The listing builds one solid part. Answer for the finished solid, in the listing's coordinates (mm). Face numbers are marked on the shaded views. A direction names the side the tool comes from. Round coordinates to 2 decimals unless told otherwise and drop trailing zeros. Loops run counter-clockwise (first coordinate to the right, second up) from the corner with the lowest first, then second, coordinate; pieces in that order, holes last. Notation, with made-up numbers: (66, 78) -> (76, 78) arc R20 ccw to (76, 108) -> close; hole circle Ø7 at (4, -2). An arc over 180 degrees is marked (long way). Write each question's results on one line, items separated by ' | '. Start each with the question number.
(1) The part is cut by section C-C (y = 2). Count the separate pieces of the cut face and the enclosed holes in it, plus the area to 3 significant figures.
(2) Flat-ended cylindrical pins translate along their axes: pin 1 (1.8 mm diameter, centred on x = 52.5, y = 2.5, fed in from -Z); pin 2 (4 mm diameter, centred on y = 10, z = 75, fed in from +X); pin 3 (6.5 mm diameter, centred on x = 52.5, y = 2, fed in from +Z). Find the tip coordinate at first contact, or state that the pin passes through.
(3) The part is cut by section B-B (z = 18.5). Determine the outline of the cut face in (x, y), plus the area to 3 significant figures.
(4) Straight lines are drawn through the part: probe 1 along Z at (x, y) = (-23.5, 1.25); probe 2 along X at (y, z) = (7.5, 64.5); probe 3 along Z at (x, y) = (53, 14.5). For each, find the intervals that lie inside material, in ascending order.
(5) Determine the mould class of the marked faces 1, 2, 3 and 4 for opening direction Z: released by +Z, released by -Z, zero draft, split by the parting line, or undercut.
(6) For the marked faces 5 and 6, determine the directions among +Z, -Z, +X, -X, +Y, -Y from which every point of the face is accessible in a straight line to the end or side of a thin tool.
(7) The part is cut by section A-A (x = 0). Determine the outline of the cut face in (y, z), plus the area to 3 significant figures.
```python
from build123d import *

# Parameters (mm, degrees)
BOSS_EXTRUDE1_DEPTH     = 16
SKETCH2_R               = 2.65
CUT_EXTRUDE1_DEPTH      = 20
CUT_EXTRUDE2_DEPTH      = 111.136478545
CUT_EXTRUDE2_DEPTH_BACK = 111.136478545
CUT_EXTRUDE3_DEPTH      = 111.136478545
CUT_EXTRUDE3_DEPTH_BACK = 111.136478545
SKETCH4_R               = 3.1
CUT_EXTRUDE4_DEPTH      = 111.136478545
CUT_EXTRUDE4_DEPTH_BACK = 6


with BuildPart() as part:
    # Sketch1 → Boss-Extrude1 (new body)
    with BuildSketch(Plane(origin=(0, 0, 0), x_dir=(1, 0, 0), z_dir=(0, 1, 0))):
        with BuildLine():
            Line((-44.75, 10.2375), (44.75, 10.2375))
            ThreePointArc((44.75, 10.2375), (57.301145366, 5.038645366), (62.5, -7.5125))
            Line((62.5, -7.5125), (62.5, -71.5125))
            ThreePointArc((62.5, -71.5125), (57.301145366, -84.063645366), (44.75, -89.2625))
            Line((44.75, -89.2625), (-44.75, -89.2625))
            ThreePointArc((-44.75, -89.2625), (-57.301145366, -84.063645366), (-62.5, -71.5125))
            Line((-62.5, -71.5125), (-62.5, -7.5125))
            ThreePointArc((-62.5, -7.5125), (-57.301145366, 5.038645366), (-44.75, 10.2375))
        make_face()
        with BuildLine():
            Line((-47.5, -7.5125), (-47.5, -71.5125))
            ThreePointArc((-47.5, -71.5125), (-46.694543648, -73.457043648), (-44.75, -74.2625))
            Line((-44.75, -74.2625), (44.75, -74.2625))
            ThreePointArc((44.75, -74.2625), (46.694543648, -73.457043648), (47.5, -71.5125))
            Line((47.5, -71.5125), (47.5, -7.5125))
            ThreePointArc((47.5, -7.5125), (46.694543648, -5.567956352), (44.75, -4.7625))
            Line((44.75, -4.7625), (-44.75, -4.7625))
            ThreePointArc((-44.75, -4.7625), (-46.694543648, -5.567956352), (-47.5, -7.5125))
        make_face(mode=Mode.SUBTRACT)
    extrude(amount=BOSS_EXTRUDE1_DEPTH)

    # Sketch2 → Cut-Extrude1 (cut)
    with BuildSketch(Plane.XY.offset(4.7625)):
        with Locations((0, 10.721875)):
            Circle(SKETCH2_R)
    extrude(amount=-CUT_EXTRUDE1_DEPTH, mode=Mode.SUBTRACT)

    # Sketch3 → Cut-Extrude2 (cut, two sides: drawn at the far end of the back side and taken through both)
    with BuildSketch(Plane(origin=(0, 0, 0), x_dir=(1, 0, 0), z_dir=(0, 1, 0)).offset(-CUT_EXTRUDE2_DEPTH_BACK)):
        with BuildLine():
            Line((-47.7, -7.5125), (-47.7, -71.5125))
            ThreePointArc((-47.7, -71.5125), (-46.835965004, -73.598465004), (-44.75, -74.4625))
            Line((-44.75, -74.4625), (44.75, -74.4625))
            ThreePointArc((44.75, -74.4625), (46.835965004, -73.598465004), (47.7, -71.5125))
            Line((47.7, -71.5125), (47.7, -7.5125))
            ThreePointArc((47.7, -7.5125), (46.835965004, -5.426534996), (44.75, -4.5625))
            Line((44.75, -4.5625), (-44.75, -4.5625))
            ThreePointArc((-44.75, -4.5625), (-46.835965004, -5.426534996), (-47.7, -7.5125))
        make_face()
        with BuildLine():
            Line((-44.75, -74.2625), (44.75, -74.2625))
            ThreePointArc((44.75, -74.2625), (46.694543648, -73.457043648), (47.5, -71.5125))
            Line((47.5, -71.5125), (47.5, -7.5125))
            ThreePointArc((47.5, -7.5125), (46.694543648, -5.567956352), (44.75, -4.7625))
            Line((44.75, -4.7625), (-44.75, -4.7625))
            ThreePointArc((-44.75, -4.7625), (-46.694543648, -5.567956352), (-47.5, -7.5125))
            Line((-47.5, -7.5125), (-47.5, -71.5125))
            ThreePointArc((-47.5, -71.5125), (-46.694543648, -73.457043648), (-44.75, -74.2625))
        make_face(mode=Mode.SUBTRACT)
    extrude(amount=CUT_EXTRUDE2_DEPTH + CUT_EXTRUDE2_DEPTH_BACK, mode=Mode.SUBTRACT)

    # Sketch4 → Cut-Extrude3 (cut, two sides: drawn at the far end of the back side and taken through both)
    with BuildSketch(Plane.XZ.offset(-CUT_EXTRUDE3_DEPTH_BACK)):
        with Locations(Location((-51.997844507, 78.760344507, 0), (0, 0, 270))):
            Circle(SKETCH4_R)
        with Locations(Location((51.997844507, 78.760344507, 0), (0, 0, 270))):
            Circle(SKETCH4_R)
        with Locations(Location((51.997844507, 0.264655493, 0), (0, 0, 270))):
            Circle(SKETCH4_R)
        with Locations(Location((-51.997844507, 0.264655493, 0), (0, 0, 270))):
            Circle(SKETCH4_R)
    extrude(amount=CUT_EXTRUDE3_DEPTH + CUT_EXTRUDE3_DEPTH_BACK, mode=Mode.SUBTRACT)

    # Sketch5 → Cut-Extrude4 (cut, two sides: drawn at the far end of the back side and taken through both)
    with BuildSketch(Plane.XZ.offset(-CUT_EXTRUDE4_DEPTH_BACK)):
        Polygon((-46.108871761, 78.760344507), (-49.053358134, 83.860344507), (-54.94233088, 83.860344507), (-57.886817253, 78.760344507), (-54.94233088, 73.660344507), (-49.053358134, 73.660344507), align=None)
        Polygon((57.886817253, 78.760344507), (54.94233088, 83.860344507), (49.053358134, 83.860344507), (46.108871761, 78.760344507), (49.053358134, 73.660344507), (54.94233088, 73.660344507), align=None)
        Polygon((57.886817253, 0.264655493), (54.94233088, 5.364655493), (49.053358134, 5.364655493), (46.108871761, 0.264655493), (49.053358134, -4.835344507), (54.94233088, -4.835344507), align=None)
        Polygon((-46.108871761, 0.264655493), (-49.053358134, 5.364655493), (-54.94233088, 5.364655493), (-57.886817253, 0.264655493), (-54.94233088, -4.835344507), (-49.053358134, -4.835344507), align=None)
    extrude(amount=CUT_EXTRUDE4_DEPTH + CUT_EXTRUDE4_DEPTH_BACK, mode=Mode.SUBTRACT)


solid = part.part
```
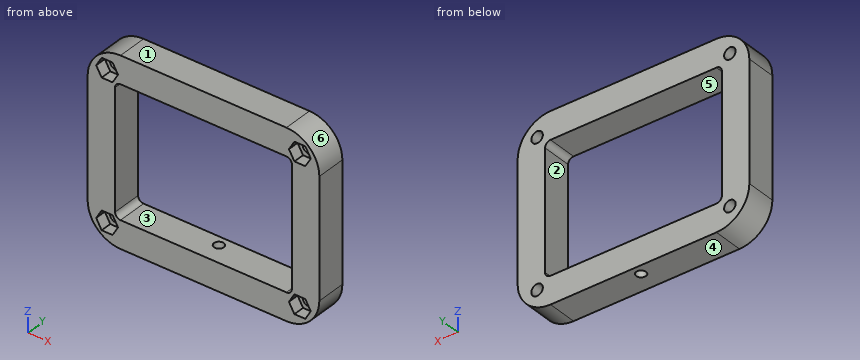
Checked values:
1) separate pieces: 1 | enclosed holes: 5 | area: 5,150 mm2
2) pin 1: stops at z = -8.86 | pin 2: stops at x = 62.44 | pin 3: stops at z = 88.68
3) outline: (-62.5, 0) -> (-47.7, 0) -> (-47.7, 16) -> (-62.5, 16) -> close; (47.7, 0) -> (62.5, 0) -> (62.5, 16) -> (47.7, 16) -> close | area: 474 mm2
4) probe 1: z = -10.24 to 4.56, 74.46 to 89.26 | probe 2: x = -62.5 to -47.7, 47.7 to 62.5 | probe 3: z = -8.2 to -2.67, 3.2 to 75.83, 81.69 to 87.23
5) face 1: released by +Z | face 2: undercut | face 3: undercut | face 4: released by -Z
6) face 5: +Y, -Y | face 6: +Z, +X, +Y, -Y
7) outline: (0, -10.24) -> (8.07, -10.24) -> (8.07, 4.56) -> (0, 4.56) -> close; (0, 74.46) -> (16, 74.46) -> (16, 89.26) -> (0, 89.26) -> close; (13.37, -10.24) -> (16, -10.24) -> (16, 4.56) -> (13.37, 4.56) -> close | area: 395 mm2
